Can you work these out from the model? Positions are in its coordinate system, mm. A direction names the side the tool comes from. Give positions to 0.01 mm unless a question says otherwise; leave off trailing zeros. Write each loop counter-clockwise with the first axis right and the second up, starting at its lowest first coordinate (ties: lowest second). Pieces come first, ordered by that corner, then holes. Notation, with made-up numbers: (-1.75, 81.25) -> (22.25, 81.25) arc R18 ccw to (22.25, 115.25) -> close; hole circle Ø8 at (60.25, 47). An arc over 180 degrees is marked (long way). Answer as CSV lines item,"result". Start each with the question number.
1. If we section it at D-D on z = -7: Write out the boundary of the cut face in (x, y), plus the area to 3 significant figures.
2. I'm going to push flat-ended pins straight in: P1, Ø1, axis at x = -28, z = -17.5, coming from the +Y side; P2, Ø4, axis at y = -7, z = 22.5, coming from the +X side; P3, Ø3, axis at x = -38.5, z = 2.5, coming from the -Y side; P4, Ø12, axis at y = -4.5, z = 7, coming from the +X side. Where does each tip first touch, or does it pass through?
3. If we section it at B-B on x = -8.5: Write out the boundary of the cut face in (y, z) (3 decimals), plus the area to 3 significant figures.
4. If we mould it in two halves opening along X, with no side actions, what happens to faces 1 (the face through (-29, -2, 0)), 2 (the face through (-8, 1, 10.795)), 3 (the face through (-23, -6, 0)), 4 (the face through (-25.958, -7.479, 21.345))? For each: pulls with the +X half, pulls with the -X half, needs draft (parallel to the pull), parting line crosses it, or undercut.
5. If we section it at A-A on z = 22.5: Write out the boundary of the cut face in (x, y).
6. If we section it at C-C on y = -7: Write out the boundary of the cut face in (x, z), plus the area to 3 significant figures.
7. On a 3-axis mill with a long thin cutter (end or side, diameter ignored), from which of +Z, -Z, +X, -X, +Y, -Y can I reach the whole of each face in a straight line? I mean faces 5 (the face through (-11, 0, 0)), 6 (the face through (-14.905, 1.268, -12.742)), 7 (the face through (-12, 2.5, 0)), 8 (the face through (-51.18, 30.23, 0.39)). Say none if no direction works.
8. I need wall thicknesses on line 1 (Z direction, x = -46.5, y = 21.5); line 2 (X direction, y = -8.5, z = 17); line 3 (Y direction, x = -2.5, z = 10). Which ranges of each line are inside material? Lowest first, please. Write a range as [from, to].
```python
from build123d import *

# Parameters (mm, degrees)
BOSS_EXTRUDE1_DEPTH = 27.5
CUT_EXTRUDE2_REACH  = 16.5
CUT_EXTRUDE3_REACH  = 33.32
SKETCH4_R           = 1.25
CUT_EXTRUDE4_REACH  = 38.642
SKETCH5_R           = 1.25


with BuildPart() as part:
    # Sketch1 → Boss-Extrude1 (new body, symmetric)
    with BuildSketch(Plane.XY):
        Polygon((0, 0), (-23, 0), (-23, -12), (-29, -12), (-29, 8), (-35.227922061, 8), (-54.319805153, 27.091883092), (-47.955844123, 33.455844123), (-23, 8.5), (-23, 2.5), (0, 2.5), align=None)
    extrude(amount=BOSS_EXTRUDE1_DEPTH, both=True)

    # Sketch3 → Cut-Extrude2 (cut, up to next)
    with BuildSketch(Plane(origin=(0, 2.5, 0), x_dir=(1, 0, 0), z_dir=(0, 1, 0)), mode=Mode.PRIVATE) as cut_extrude2_sk1:
        with BuildLine():
            Line((-13, -10.795), (-3, -10.795))
            ThreePointArc((-3, -10.795), (-1.095, -12.7), (-3, -14.605))
            Line((-3, -14.605), (-13, -14.605))
            ThreePointArc((-13, -14.605), (-14.905, -12.7), (-13, -10.795))
        make_face()
    cut_extrude2_tool1 = extrude(cut_extrude2_sk1.sketch, amount=-CUT_EXTRUDE2_REACH, mode=Mode.PRIVATE) & part.part
    add(cut_extrude2_tool1.solids().sort_by_distance((-8, 2.5, 12.7))[0], mode=Mode.SUBTRACT)
    # Sketch3 → Cut-Extrude2 (cut, up to next)
    with BuildSketch(Plane(origin=(0, 2.5, 0), x_dir=(1, 0, 0), z_dir=(0, 1, 0)), mode=Mode.PRIVATE) as cut_extrude2_sk2:
        with BuildLine():
            Line((-13, 10.795), (-3, 10.795))
            ThreePointArc((-3, 10.795), (-1.095, 12.7), (-3, 14.605))
            Line((-3, 14.605), (-13, 14.605))
            ThreePointArc((-13, 14.605), (-14.905, 12.7), (-13, 10.795))
        make_face()
    cut_extrude2_tool2 = extrude(cut_extrude2_sk2.sketch, amount=-CUT_EXTRUDE2_REACH, mode=Mode.PRIVATE) & part.part
    add(cut_extrude2_tool2.solids().sort_by_distance((-8, 2.5, -12.7))[0], mode=Mode.SUBTRACT)

    # Sketch4 → Cut-Extrude3 (cut, up to next)
    with BuildSketch(Plane(origin=(-23, 0, 0), x_dir=(0, 0, -1), z_dir=(1, 0, 0)), mode=Mode.PRIVATE) as cut_extrude3_sk1:
        with Locations((-22.5, -7)):
            Circle(SKETCH4_R)
    cut_extrude3_tool1 = extrude(cut_extrude3_sk1.sketch, amount=-CUT_EXTRUDE3_REACH, mode=Mode.PRIVATE) & part.part
    add(cut_extrude3_tool1.solids().sort_by_distance((-23, -7, 22.5))[0], mode=Mode.SUBTRACT)
    # Sketch4 → Cut-Extrude3 (cut, up to next)
    with BuildSketch(Plane(origin=(-23, 0, 0), x_dir=(0, 0, -1), z_dir=(1, 0, 0)), mode=Mode.PRIVATE) as cut_extrude3_sk2:
        with Locations((22.5, -7)):
            Circle(SKETCH4_R)
    cut_extrude3_tool2 = extrude(cut_extrude3_sk2.sketch, amount=-CUT_EXTRUDE3_REACH, mode=Mode.PRIVATE) & part.part
    add(cut_extrude3_tool2.solids().sort_by_distance((-23, -7, -22.5))[0], mode=Mode.SUBTRACT)

    # Sketch5 → Cut-Extrude4 (cut, up to next)
    with BuildSketch(Plane(origin=(-7.25, -7.25, 0), x_dir=(0, 0, -1), z_dir=(0.707106781, 0.707106781, 0)), mode=Mode.PRIVATE) as cut_extrude4_sk1:
        with Locations((-25, 47.566756826)):
            Circle(SKETCH5_R)
    cut_extrude4_tool1 = extrude(cut_extrude4_sk1.sketch, amount=-CUT_EXTRUDE4_REACH, mode=Mode.PRIVATE) & part.part
    add(cut_extrude4_tool1.solids().sort_by_distance((-40.884776, 26.384776, 25))[0], mode=Mode.SUBTRACT)
    # Sketch5 → Cut-Extrude4 (cut, up to next)
    with BuildSketch(Plane(origin=(-7.25, -7.25, 0), x_dir=(0, 0, -1), z_dir=(0.707106781, 0.707106781, 0)), mode=Mode.PRIVATE) as cut_extrude4_sk2:
        with Locations((25, 47.566756826)):
            Circle(SKETCH5_R)
    cut_extrude4_tool2 = extrude(cut_extrude4_sk2.sketch, amount=-CUT_EXTRUDE4_REACH, mode=Mode.PRIVATE) & part.part
    add(cut_extrude4_tool2.solids().sort_by_distance((-40.884776, 26.384776, -25))[0], mode=Mode.SUBTRACT)


solid = part.part
```
Computed values:
1,outline,"(-54.32, 27.09) -> (-35.23, 8) -> (-29, 8) -> (-29, -12) -> (-23, -12) -> (-23, 0) -> (0, 0) -> (0, 2.5) -> (-23, 2.5) -> (-23, 8.5) -> (-47.96, 33.46) -> close"
1,area,"461 mm2"
2,P1,"stops at y = 14"
2,P2,"stops at x = -23"
2,P3,"stops at y = 9.77"
2,P4,"stops at x = 0"
3,outline,"(0, -27.5) -> (2.5, -27.5) -> (2.5, -14.605) -> (0, -14.605) -> close; (0, -10.795) -> (2.5, -10.795) -> (2.5, 10.795) -> (0, 10.795) -> close; (0, 14.605) -> (2.5, 14.605) -> (2.5, 27.5) -> (0, 27.5) -> close"
3,area,"118 mm2"
4,face 1,"pulls with the -X half"
4,face 2,"undercut"
4,face 3,"pulls with the +X half"
4,face 4,"needs draft"
5,outline,"(-54.32, 27.09) -> (-35.23, 8) -> (-29, 8) -> (-29, -5.75) -> (-23, -5.75) -> (-23, 0) -> (0, 0) -> (0, 2.5) -> (-23, 2.5) -> (-23, 8.5) -> (-47.96, 33.46) -> close; (-29, -12) -> (-23, -12) -> (-23, -8.25) -> (-29, -8.25) -> close"
6,outline,"(-29, -27.5) -> (-23, -27.5) -> (-23, -23.75) -> (-29, -23.75) -> close; (-29, -21.25) -> (-23, -21.25) -> (-23, 21.25) -> (-29, 21.25) -> close; (-29, 23.75) -> (-23, 23.75) -> (-23, 27.5) -> (-29, 27.5) -> close"
6,area,"300 mm2"
7,face 5,"+Z, -Z, +X, -Y"
7,face 6,"+Y, -Y"
7,face 7,"+Z, -Z, +X, +Y"
7,face 8,"+Z, -Z, -X, +Y"
8,line 1,"z = [-27.5, -26.14], [-23.86, 23.86], [26.14, 27.5]"
8,line 2,"x = [-29, -23]"
8,line 3,"y = [0, 2.5]"
